Geometry: final body of the model. Coordinates: model frame, mm. A direction names the side the tool comes from. Coordinates: 2 decimals unless noted, no trailing zeros. Write each loop counter-clockwise with the first axis right and the second up, starting at its lowest first coordinate (ties: lowest second). Pieces come first, ordered by that corner, then holes. Notation, with made-up numbers: (-22.5, -29.5) -> (0.5, -29.5) arc R15 cw to (0.5, -11.5) -> close; hole circle Ø10 at (81, 40). An arc over 180 degrees is marked (long way). Answer as a JSON object with one key per item and string values. Group by question number.
```python
from build123d import *

# Parameters (mm, degrees)
F1_DEPTH = 431.8
F3_D     = 9.525


with BuildPart() as f1:
    # F0 (on Top) → F1 (new body)
    with BuildSketch(Plane.XY):
        with BuildLine():
            ThreePointArc((-10.3378, 12.7), (-12.008128, 12.008128), (-12.7, 10.3378))
            Line((-12.7, 10.3378), (-12.7, -10.3378))
            ThreePointArc((-12.7, -10.3378), (-12.008128, -12.008128), (-10.3378, -12.7))
            Line((-10.3378, -12.7), (10.3378, -12.7))
            ThreePointArc((10.3378, -12.7), (12.008128, -12.008128), (12.7, -10.3378))
            Line((12.7, -10.3378), (12.7, 10.3378))
            ThreePointArc((12.7, 10.3378), (12.008128, 12.008128), (10.3378, 12.7))
            Line((10.3378, 12.7), (-10.3378, 12.7))
        make_face()
        with BuildLine():
            Line((-8.8138, 10.3378), (8.8138, 10.3378))
            ThreePointArc((8.8138, 10.3378), (9.891431, 9.891431), (10.3378, 8.8138))
            Line((10.3378, 8.8138), (10.3378, -8.8138))
            ThreePointArc((10.3378, -8.8138), (9.891431, -9.891431), (8.8138, -10.3378))
            Line((8.8138, -10.3378), (-8.8138, -10.3378))
            ThreePointArc((-8.8138, -10.3378), (-9.891431, -9.891431), (-10.3378, -8.8138))
            Line((-10.3378, -8.8138), (-10.3378, 8.8138))
            ThreePointArc((-10.3378, 8.8138), (-9.891431, 9.891431), (-8.8138, 10.3378))
        make_face(mode=Mode.SUBTRACT)
    extrude(amount=F1_DEPTH)

    # F3 (through all)
    with Locations(Plane.YZ.offset(12.7)):
        with Locations((0, 247.65), (0, 184.15)):
            Hole(F3_D / 2)


solid = f1.part
```
Item 1: Section D-D on z = 199.5. Output: boundary loops of the cut face in (x, y), then the cut area to 3 significant figures.
Item 2: Set-up query: faces 4 (the flat face through (-12.7, 0, 213)), 5 (the flat face through (0, -10.338, 213)). Return all of +Z, -Z, +X, -X, +Y, -Y with unobstructed straight access to the full face (end or side cutting, diameter ignored); none if empty.
Item 3: Ray query, L1, parallel to Z at x = 11.35, y = 0; L2, parallel to X at y = 8.5, z = 398. Return the intervals inside material, ascending. Write a range as [from, to].
Item 4: Mould query, pull axis X, two halves, no side actions, for faces 1 (the cylindrical face through (11.5, 1.03, 179.5)), 2 (the flat face through (12.7, 0, 213)), 3 (the flat face through (0, 10.338, 213)). Classes: +X half, -X half, draft (parallel to the pull), parting line (faces both ways), or undercut.
Item 5: Contact query for a flat-ended pin moving along its axis: pin 1 (7.5 mm diameter, centred on y = 0, z = 247.65, fed in from +X). Output: stop coordinate, or through.
Item 6: Section B-B on z = 247.65. Output: boundary loops of the cut face in (x, y), then the cut area to 3 significant figures.
Item 7: Section C-C on y = 0. Output: boundary loops of the cut face in (x, z).
Item 8: Section A-A on x = -2.25. Output: boundary loops of the cut face in (y, z), then the cut area to 3 significant figures.
Answer sheet:
{
 "1": {"outline": "(-12.7, -10.34) arc R2.36 ccw to (-10.34, -12.7) -> (10.34, -12.7) arc R2.36 ccw to (12.7, -10.34) -> (12.7, 10.34) arc R2.36 ccw to (10.34, 12.7) -> (-10.34, 12.7) arc R2.36 ccw to (-12.7, 10.34) -> close; hole (-10.34, -8.81) arc R1.52 ccw to (-8.81, -10.34) -> (8.81, -10.34) arc R1.52 ccw to (10.34, -8.81) -> (10.34, 8.81) arc R1.52 ccw to (8.81, 10.34) -> (-8.81, 10.34) arc R1.52 ccw to (-10.34, 8.81) -> close", "area": "215 mm^2"},
 "2": {"face 4": "+Z, -Z, -X, +Y, -Y", "face 5": "+Z, -Z"},
 "3": {"L1": "z = [0, 179.39], [188.91, 242.89], [252.41, 431.8]", "L2": "x = [-12.7, -10.34], [10.34, 12.7]"},
 "4": {"face 1": "draft", "face 2": "+X half", "face 3": "undercut"},
 "5": {"pin 1": "passes through"},
 "6": {"outline": "(-12.7, -10.34) arc R2.36 ccw to (-10.34, -12.7) -> (10.34, -12.7) arc R2.36 ccw to (12.7, -10.34) -> (12.7, -4.76) -> (10.34, -4.76) -> (10.34, -8.81) arc R1.52 cw to (8.81, -10.34) -> (-8.81, -10.34) arc R1.52 cw to (-10.34, -8.81) -> (-10.34, -4.76) -> (-12.7, -4.76) -> close; (-12.7, 4.76) -> (-10.34, 4.76) -> (-10.34, 8.81) arc R1.52 cw to (-8.81, 10.34) -> (8.81, 10.34) arc R1.52 cw to (10.34, 8.81) -> (10.34, 4.76) -> (12.7, 4.76) -> (12.7, 10.34) arc R2.36 ccw to (10.34, 12.7) -> (-10.34, 12.7) arc R2.36 ccw to (-12.7, 10.34) -> close", "area": "170 mm^2"},
 "7": {"outline": "(-12.7, 0) -> (-10.34, 0) -> (-10.34, 179.39) -> (-12.7, 179.39) -> close; (-12.7, 188.91) -> (-10.34, 188.91) -> (-10.34, 242.89) -> (-12.7, 242.89) -> close; (-12.7, 252.41) -> (-10.34, 252.41) -> (-10.34, 431.8) -> (-12.7, 431.8) -> close; (10.34, 0) -> (12.7, 0) -> (12.7, 179.39) -> (10.34, 179.39) -> close; (10.34, 188.91) -> (12.7, 188.91) -> (12.7, 242.89) -> (10.34, 242.89) -> close; (10.34, 252.41) -> (12.7, 252.41) -> (12.7, 431.8) -> (10.34, 431.8) -> close"},
 "8": {"outline": "(-12.7, 0) -> (-10.34, 0) -> (-10.34, 431.8) -> (-12.7, 431.8) -> close; (10.34, 0) -> (12.7, 0) -> (12.7, 431.8) -> (10.34, 431.8) -> close", "area": "2,040 mm^2"}
}
